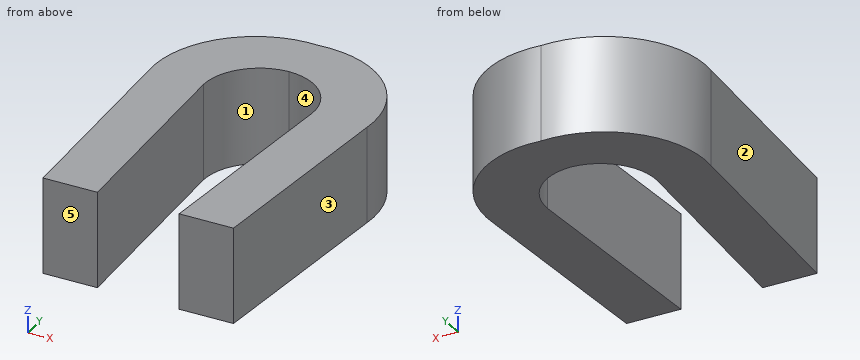
```python
from build123d import *

# Parameters (mm, degrees)
BOSS_EXTRUDE1_DEPTH = 3.5


with BuildPart() as part:
    # Sketch1 → Boss-Extrude1 (new body)
    with BuildSketch(Plane.XY):
        with BuildLine():
            Line((-2, 4), (-1.5, -4))
            Line((-1.5, -4), (-3.5, -4))
            Line((-3.5, -4), (-4, 4))
            ThreePointArc((-4, 4), (-2.950434096, 6.97104187), (0, 8.077214108))
            ThreePointArc((0, 8.077214108), (2.950434096, 6.97104187), (4, 4))
            Line((4, 4), (3.5, -4))
            Line((3.5, -4), (1.5, -4))
            Line((1.5, -4), (2, 4))
            ThreePointArc((2, 4), (1.430965913, 5.453553122), (0, 6.077214108))
            ThreePointArc((0, 6.077214108), (-1.430965913, 5.453553122), (-2, 4))
        make_face()
    extrude(amount=BOSS_EXTRUDE1_DEPTH)


solid = part.part
```
Can you work these out from the model? Positions are in its coordinate system, mm. Face numbers are marked on the shaded views. A direction names the side the tool comes from. Coordinates: 2 decimals unless noted, no trailing zeros. Loops run counter-clockwise (first coordinate to the right, second up) from the corner with the lowest first, then second, coordinate; pieces in that order, holes last.
1) Imagine slicing it at A-A on y = 4.5. List the corners of the cut face in (x, z) for me, plus the area to 3 significant figures.
2) Thinking about a two-plate mould opening in X: for the marked faces 3, 4 and 5, which applies, pulls with the +X half, pulls with the -X half, needs draft (parallel to the pull), parting line crosses it, or undercut?
3) Imagine slicing it at C-C on z = 2.5. List the corners of the cut face in (x, y) for me, plus the area to 3 significant figures.
4) Which directions (+Z, -Z, +X, -X, +Y, -Y) give clear straight access to the entire face, cutting with the end or side of a thin tool? Please do the marked faces 1 and 2.
5) I need wall thicknesses on probe 1 along X at (y, z) = (3.75, 2.45); probe 2 along X at (y, z) = (3, 2.85); probe 3 along X at (y, z) = (7.5, 1). Which ranges of each line are inside material? Lowest first, please.
6) Imagine slicing it at B-B on x = 1.75. List the corners of the cut face in (y, z) for me, plus the area to 3 significant figures.
7) For pin 1 (1 mm diameter, centred on x = -1.5, z = 0.5, fed in from +Y); pin 2 (1.5 mm diameter, centred on y = 6.5, z = 2, fed in from +X); pin 3 (1 mm diameter, centred on y = 3, z = 1.5, fed in from +X), each with a flat end and sliding along its axis, tell me the tip position at first contact or that it passes through.
8) Imagine slicing it at D-D on x = -1.25. List the corners of the cut face in (y, z) for me.
Completed:
1. outline: (-4.01, 0) - (-1.95, 0) - (-1.95, 3.5) - (-4.01, 3.5) - close; (1.95, 0) - (4.01, 0) - (4.01, 3.5) - (1.95, 3.5) - close
1. area: 14.5 mm2
2. face 3: pulls with the +X half
2. face 4: undercut
2. face 5: needs draft
3. outline: (-4, 4) - (-3.5, -4) - (-1.5, -4) - (-2, 4) arc R2.04 cw to (0, 6.08) arc R2.04 cw to (2, 4) - (1.5, -4) - (3.5, -4) - (4, 4) arc R3.73 ccw to (0, 8.08) arc R3.73 ccw to start
3. area: 52.3 mm2
4. face 1: +Z, -Z
4. face 2: +Z, -Z, -X, -Y
5. probe 1: x = -3.98 to -1.98, 1.98 to 3.98
5. probe 2: x = -3.94 to -1.94, 1.94 to 3.94
5. probe 3: x = -2.3 to 2.3
6. outline: (-4, 0) - (0, 0) - (0, 3.5) - (-4, 3.5) - close; (5.02, 0) - (7.79, 0) - (7.79, 3.5) - (5.02, 3.5) - close
6. area: 23.7 mm2
7. pin 1: stops at y = 8.02
7. pin 2: stops at x = 3.75
7. pin 3: stops at x = 3.97
8. outline: (5.62, 0) - (7.96, 0) - (7.96, 3.5) - (5.62, 3.5) - close
